Verification items for the finished model (mm, model axes). Round coordinates to 2 decimals unless told otherwise and drop trailing zeros. Loops run counter-clockwise (first coordinate to the right, second up) from the corner with the lowest first, then second, coordinate; pieces in that order, holes last. Notation, with made-up numbers: (32.25, 58) - (71.25, 58) arc R19 cw to (71.25, 74) - close; hole circle Ø10 at (-35, 14). An arc over 180 degrees is marked (long way). Use CSV: the item, a comma, the result in double quotes.
```python
from build123d import *

# Parameters (mm, degrees)
CROQUIS1_R              = 4
CROQUIS1_R_2            = 2.5
SALIENTE_EXTRUIR1_DEPTH = 11
CROQUIS2_R              = 1.5
CORTAR_EXTRUIR2_DEPTH   = 2
CROQUIS3_R              = 3.5


with BuildPart() as part:
    # Croquis1 → Saliente-Extruir1 (new body)
    with BuildSketch(Plane(origin=(0, 0, 0), x_dir=(1, 0, 0), z_dir=(0, 1, 0))):
        Circle(CROQUIS1_R)
        Circle(CROQUIS1_R_2, mode=Mode.SUBTRACT)
    extrude(amount=SALIENTE_EXTRUIR1_DEPTH)

    # Croquis2 → Cortar-Extruir2 (cut)
    with BuildSketch(Plane(origin=(4, 0, 0), x_dir=(0, 0, -1), z_dir=(1, 0, 0))):
        with Locations((0, 2.5)):
            Circle(CROQUIS2_R)
    extrude(amount=-CORTAR_EXTRUIR2_DEPTH, mode=Mode.SUBTRACT)

    # Croquis3 → Cortar-Revoluci_n2 (revolve, cut)
    with BuildSketch(Plane.XY):
        with Locations((6.75, 7.5)):
            Circle(CROQUIS3_R)
    revolve(axis=Axis((0, 0, 0), (0, 1, 0)), mode=Mode.SUBTRACT)


solid = part.part
```
1) Mould release check, pull along Y, two halves, no side actions. Record for faces 1 (the face through (-0.867, 10.323, 3.905)), 2 (the face through (2, 11, -2)), 3 (the face through (3.01, 2.95, -1.43)): +Y half, -Y half, draft (parallel to the pull), parting line (faces both ways), or undercut.
Returned:
face 1,"draft"
face 2,"+Y half"
face 3,"undercut"
2) Thickness scan on probe 1 along Y at (x, z) = (3.55, 0); probe 2 along Y at (x, z) = (2.9, 0); probe 3 along Y at (x, z) = (3.5, -0.75). Record the ranges inside material, lowest first. Write a range as [from, to].
Returned:
probe 1,"y = [0, 1], [4, 6.08], [8.92, 11]"
probe 2,"y = [0, 1], [4, 11]"
probe 3,"y = [0, 1.2], [3.8, 6.02], [8.98, 11]"
3) Cross-section at C-C, the plane y = 7. Record the cut outline in (x, z).
Returned:
outline,"circle Ø6.57 at (0, 0); hole circle Ø5 at (0, 0)"
4) Cross-section at D-D, the plane y = 2.5. Record the cut outline in (x, z).
Returned:
outline,"(2, -1.5) arc R2.5 cw (long way) to (2, 1.5) - (3.71, 1.5) arc R4 ccw (long way) to (3.71, -1.5) - close"
5) Cross-section at A-A, the plane x = 0. Record the cut outline in (y, z), then the cut area to 3 significant figures.
Returned:
outline,"(0, -4) - (5.33, -4) arc R3.5 cw to (9.67, -4) - (11, -4) - (11, -2.5) - (0, -2.5) - close; (0, 2.5) - (11, 2.5) - (11, 4) - (9.67, 4) arc R3.5 cw to (5.33, 4) - (0, 4) - close"
area,"28.6 mm²"
6) Cross-section at B-B, the plane z = 0. Record the cut outline in (x, y).
Returned:
outline,"(-4, 0) - (-2.5, 0) - (-2.5, 11) - (-4, 11) - (-4, 9.67) arc R3.5 cw to (-4, 5.33) - close; (2.5, 0) - (4, 0) - (4, 1) - (2.5, 1) - close; (2.5, 4) - (4, 4) - (4, 5.33) arc R3.5 cw to (4, 9.67) - (4, 11) - (2.5, 11) - close"
7) Gauge pin test, flat end, axial feed: pin 1 Ø1.5 at (y, z) = (5.5, -2) entering from -X. Record the tip position at first contact, or that the pin passes through.
Returned:
pin 1,"stops at x = -3.79"
